Read the model definition and answer for the solid it produces. Units are mm, in the model's axes. Face numbers are marked on the shaded views. A direction names the side the tool comes from. Coordinates: 2 decimals unless noted, no trailing zeros. Loops run counter-clockwise (first coordinate to the right, second up) from the corner with the lowest first, then second, coordinate; pieces in that order, holes last. Notation, with made-up numbers: (29.25, -10) - (62.25, -10) arc R18 cw to (62.25, 0) - close; hole circle Ø5 at (69.25, 73.5). An arc over 180 degrees is marked (long way). Use one line per item in the form item = value. Start each with the question number.
1) A cutting plane is placed at A-A (y = 0). Give the vertices of the cut face in (x, z), and give its area (3 significant figures).
2) A cutting plane is placed at B-B (z = 43). Give the vertices of the cut face in (x, y), and give its area (3 significant figures).
3) Consider line 1 (Y direction, x = 0, z = 36); line 2 (Z direction, x = 7, y = 13.5); line 3 (Z direction, x = 0, y = -11.75). Determine where each line is inside the solid, lowest interval first.
4) The mould has two halves that part along X. Classify the marked faces 3, 4, 5 and 6: released by +X, released by -X, zero draft, split by the parting line, or undercut.
5) A cutting plane is placed at C-C (z = 17.5). Give the vertices of the cut face in (x, y).
6) Each of these flat-tipped pins is pushed along its axis until it touches: P1, Ø5.5, axis at x = 0, z = 43, coming from the -Y side; P2, Ø5, axis at x = -0.5, z = 44.5, coming from the +Y side; P3, Ø3, axis at y = -13.5, z = 47, coming from the -X side; P4, Ø10, axis at y = 2.5, z = 34.5, coming from the -X side. Where does it stop, or does it pass through?
7) Which of the six approach directions +Z, -Z, +X, -X, +Y, -Y give full straight-line access (tool end or side, diameter ignored) to the marked faces 1 and 2?
8) A cutting plane is placed at D-D (y = -19.5). Give the vertices of the cut face in (x, z), and give its area (3 significant figures).
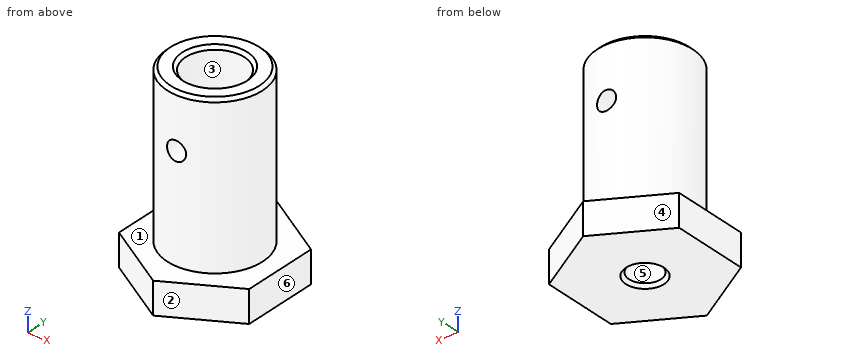
Autodesk Inventor part; units mm, degrees
ref_plane "YZ Plane" through (0, 0, 0) normal (1, 0, 0) x (0, 1, 0)
ref_plane "XZ Plane" through (0, 0, 0) normal (0, 1, 0) x (-1, 0, 0)
ref_plane "XY Plane" through (0, 0, 0) normal (0, 0, 1) x (1, 0, 0)
sketch "Эскиз1" plane through (0, 0, 0) normal (0, 0, 1) x (1, 0, 0)
  line L0 (0, 23.6714) -> (20.5, 11.8357)
  line L1 (20.5, 11.8357) -> (20.5, -11.8357)
  line L2 (20.5, -11.8357) -> (0, -23.6714)
  line L3 (0, -23.6714) -> (-20.5, -11.8357)
  line L4 (-20.5, -11.8357) -> (-20.5, 11.8357)
  line L5 (-20.5, 11.8357) -> (0, 23.6714)
  point P0 (0, 0)
  point P1 (0, 0)
  dimension "d27" = 41
extrude "Выдавливание1" add sketch "Эскиз1" along normal blind 10
sketch "Эскиз2" plane through (0, 0, 10) normal (0, 0, 1) x (1, 0, 0)
  circle A0 centre (0, 0) radius 15
  dimension "d3" = 30
extrude "Выдавливание2" add sketch "Эскиз2" along normal blind 50
sketch "Эскиз3" plane through (0, 0, 60) normal (0, 0, 1) x (1, 0, 0)
  point P0 (0, 0)
  point P1 (0, 0)
hole "Отверстие1" at (0, 0, 60) direction (0, 0, -1) diameter 18.5 depth 30 tip angle 120
sketch "Эскиз4" plane through (0, 0, 0) normal (0, 0, -1) x (-1, 0, 0)
  point P0 (0, 0)
  point P1 (0, 0)
hole "Отверстие2" at (0, 0, 0) direction (0, 0, 1) diameter 10 end through all
sketch "Эскиз5" plane through (0, 0, 0) normal (0, 1, 0) x (-1, 0, 0)
  circle A0 centre (0, 43) radius 3
  line L0 (15, 60) -> (-15, 60)
  point P0 (0, 0)
  dimension "d20" = 6
  dimension "d21" = 17
extrude "Выдавливание3" cut sketch "Эскиз5" along normal through all both and the other way through all
chamfer "Фаска1" distance 1 angle 45 3 edges at (0, 9.25, 60) (-15, 0, 60) (0, -5, 0)
properties part number "И7-22"
Found:
q1.outline = (-20.5, 0) - (-6, 0) - (-5, 1) - (-5, 27.55) - (-9.25, 30) - (-9.25, 59) - (-10.25, 60) - (-14, 60) - (-15, 59) - (-15, 10) - (-20.5, 10) - close; (5, 1) - (6, 0) - (20.5, 0) - (20.5, 10) - (15, 10) - (15, 59) - (14, 60) - (10.25, 60) - (9.25, 59) - (9.25, 30) - (5, 27.55) - close
q1.area = 1,040 mm^2
q2.outline = (-3, -14.7) - (-3, -8.75) arc R9.25 cw to (-3, 8.75) - (-3, 14.7) arc R15 ccw to start; (3, -14.7) arc R15 ccw to (3, 14.7) - (3, 8.75) arc R9.25 cw to (3, -8.75) - close
q2.area = 368 mm^2
q3.line_1 = -15 to -9.25, 9.25 to 15
q3.line_2 = 0 to 10
q3.line_3 = 0 to 40, 46 to 60
q4.face_3 = undercut
q4.face_4 = released by -X
q4.face_5 = undercut
q4.face_6 = released by +X
q5.outline = circle Ø30 at (0, 0); hole circle Ø10 at (0, 0)
q6.P1 = through
q6.P2 = 15
q6.P3 = -9
q6.P4 = -15
q7.face_1 = +Z
q7.face_2 = +Z, -Z, +X, -Y
q8.outline = (-7.23, 0) - (7.23, 0) - (7.23, 10) - (-7.23, 10) - close
q8.area = 145 mm^2
